```python
from build123d import *

# Parameters (mm, degrees)
SKETCH_1_W          = 30
SKETCH_1_H          = 20
EXTRUDE_1_DEPTH     = 10
SKETCH_2_R          = 2.5
CUT_EXTRUDE_1_DEPTH = 21.615528128
SKETCH_3_W          = 30
SKETCH_3_H          = 6
EXTRUDE_2_DEPTH     = 30
SKETCH_4_R          = 7.5
CUT_EXTRUDE_2_DEPTH = 30
FILLET_1_R          = 10
FILLET_2_R          = 10
FILLET_3_R          = 1
FILLET_4_R          = 1


with BuildPart() as part:
    # 草图1 → 凸台-拉伸1 (new body)
    with BuildSketch(Plane.XY):
        Rectangle(SKETCH_1_W, SKETCH_1_H)
    extrude(amount=EXTRUDE_1_DEPTH)

    # 草图2 → 切除-拉伸1 (cut, through all)
    with BuildSketch(Plane.XY.offset(10)):
        with Locations((-10, 0)):
            Circle(SKETCH_2_R)
        with Locations((10, 0)):
            Circle(SKETCH_2_R)
    extrude(amount=-CUT_EXTRUDE_1_DEPTH, mode=Mode.SUBTRACT)

    # 草图3 → 凸台-拉伸2 (add)
    with BuildSketch(Plane.XY.offset(10)):
        with Locations((0, -7)):
            Rectangle(SKETCH_3_W, SKETCH_3_H)
    extrude(amount=EXTRUDE_2_DEPTH)

    # 草图4 → 切除-拉伸2 (cut)
    with BuildSketch(Plane.XZ.offset(10)):
        with Locations(Location((0, 25, 0), (0, 0, 270))):
            Circle(SKETCH_4_R)
    extrude(amount=-CUT_EXTRUDE_2_DEPTH, mode=Mode.SUBTRACT)

    # 圆角1
    fillet_1_edges = [part.edges().sort_by_distance(p)[0] for p in [
        (-15, -7, 40),
        (15, -7, 40),
    ]]
    fillet(fillet_1_edges, radius=FILLET_1_R)

    # 圆角2
    fillet_2_edges = [part.edges().sort_by_distance(p)[0] for p in [
        (-15, 10, 5),
        (15, 10, 5),
    ]]
    fillet(fillet_2_edges, radius=FILLET_2_R)

    # 圆角3
    fillet_3_edges = [part.edges().sort_by_distance(p)[0] for p in [
        (0, -10, 40),
        (0, -10, 0),
        (15, -10, 15),
        (-15, -10, 15),
        (12.071067812, -10, 37.071067812),
        (-12.071067812, -10, 37.071067812),
        (15, -5, 0),
        (0, 10, 0),
        (-15, -5, 0),
        (-12.071067812, 7.071067812, 0),
        (12.071067812, 7.071067812, 0),
    ]]
    fillet(fillet_3_edges, radius=FILLET_3_R)

    # 圆角4
    fillet_4_edges = [part.edges().sort_by_distance(p)[0] for p in [
        (15, -2, 10),
        (0, -4, 40),
        (-15, -4, 20),
        (15, -4, 20),
        (12.071067812, -4, 37.071067812),
        (-12.071067812, -4, 37.071067812),
        (0, 10, 10),
        (-15, -2, 10),
        (-12.071067812, 7.071067812, 10),
        (12.071067812, 7.071067812, 10),
    ]]
    fillet(fillet_4_edges, radius=FILLET_4_R)


solid = part.part
```
The model under review builds one solid part; all positions refer to its coordinate system, in mm. A direction names the side the tool comes from. Round coordinates to 2 decimals unless told otherwise and drop trailing zeros. Loops run counter-clockwise (first coordinate to the right, second up) from the corner with the lowest first, then second, coordinate; pieces in that order, holes last. Notation, with made-up numbers: M -19.75,-5 L -15.75,-5 A13 ccw -15.75,20 Z; hole C 23.5,47.25 d8. An arc over 180 degrees is marked long. Answer as a JSON object with one key per item and string values.
(1) Take a section at C-C on z = 16. Give the boundary of the cut face in (x, y).
Resolved:
{"outline": "M -15,-9 A1 ccw -14,-10 L 14,-10 A1 ccw 15,-9 L 15,-5 A1 ccw 14,-4 L -14,-4 A1 ccw -15,-5 Z"}
(2) Take a section at B-B on x = 0. Give the boundary of the cut face in (y, z), and give its area (3 significant figures).
Resolved:
{"outline": "M -10,1 A1 ccw -9,0 L 9,0 A1 ccw 10,1 L 10,9 A1 ccw 9,10 L -4,10 L -4,17.5 L -10,17.5 Z; M -10,32.5 L -4,32.5 L -4,39 A1 ccw -5,40 L -9,40 A1 ccw -10,39 Z", "area": "289 mm²"}
(3) To check wall thickness, follow line 1 along X through (y, z) = (-8.7, 25); line 2 along Y through (x, z) = (-1, 12); line 3 along X through (y, z) = (2.25, 2). State the ranges of each line that lie inside material, in increasing order.
Resolved:
{"line 1": "-15 to -7.5, 7.5 to 15", "line 2": "-10 to -4", "line 3": "-14.74 to -11.09, -8.91 to 8.91, 11.09 to 14.74"}
(4) Tool access review of faces 4 (the flat face through (-15, -6, 12)), 5 (the cylindrical face through (-14.699, -4.285, 19.647)), 6 (the flat face through (0, 3, 10)), 7 (the cylindrical face through (14.699, -4.285, 19.353)), 8 (the cylindrical face through (-14.699, -9.715, 15.703)): name each direction out of +Z, -Z, +X, -X, +Y, -Y from which nothing blocks a thin tool from reaching the whole face with its end or side.
Resolved:
{"face 4": "+Z, -Z, -X, +Y, -Y", "face 5": "+Z, -X, +Y", "face 6": "+Z, +X, -X, +Y", "face 7": "+Z, +X, +Y", "face 8": "+Z, -Z, -X, -Y"}
(5) Draft analysis for pull direction Y (two halves, no side actions). For faces 1 (the cylindrical face through (0.07, -4.285, 39.699)), 2 (the cylindrical face through (7.5, 0.1, 5.1)), 3 (the cylindrical face through (-12.15, -6.97, 36.99)), state which applies: released by +Y, released by -Y, zero draft, split by the parting line, or undercut.
Resolved:
{"face 1": "released by +Y", "face 2": "undercut", "face 3": "zero draft"}
(6) Clearance check with flat-ended pins moving along their axes: P1, Ø4, axis at x = 0, z = 11.5, coming from the +Y side; P2, Ø14, axis at x = -2, z = 20.5, coming from the +Y side; P3, Ø1, axis at y = 3.5, z = 9, coming from the +X side. State where each tip first meets the part, or that it passes through.
Resolved:
{"P1": "y = 9.87", "P2": "y = -4", "P3": "x = 14.54"}
(7) Take a section at A-A on z = 25. Give the boundary of the cut face in (x, y).
Resolved:
{"outline": "M -15,-9 A1 ccw -14,-10 L -7.5,-10 L -7.5,-4 L -14,-4 A1 ccw -15,-5 Z; M 7.5,-10 L 14,-10 A1 ccw 15,-9 L 15,-5 A1 ccw 14,-4 L 7.5,-4 Z"}
(8) Take a section at D-D on y = -3. Give the boundary of the cut face in (x, z).
Resolved:
{"outline": "M -15,1 A1 ccw -14,0 L 14,0 A1 ccw 15,1 L 15,9 A1 ccw 14,10 L -14,10 A1 ccw -15,9 Z"}
